For this review, take the finished solid that the model builds, in its own axes (mm). Face numbers are marked on the shaded views. A direction names the side the tool comes from. Round coordinates to 2 decimals unless told otherwise and drop trailing zeros. Order: outer loops, then holes, each group sorted by start corner. A loop starts at its lowest first (then second) coordinate and runs counter-clockwise, first axis right, second up. Notation, with made-up numbers: (1, -13.75) - (27, -13.75) arc R25 ccw to (27, 8.25) - close; hole circle Ø8 at (-13, 57). An arc over 180 degrees is marked (long way). Write each question's results on one line, items separated by ' | '. Start each with the question number.
(1) Draft analysis for pull direction X (two halves, no side actions). For the marked faces 5, 6 and 7, state which applies: pulls with the +X half, pulls with the -X half, needs draft (parallel to the pull), parting line crosses it, or undercut.
(2) For L1, parallel to Y at x = 5.5, z = 1.75; L2, parallel to Z at x = -11.5, y = -2; L3, parallel to Y at x = 11.7, z = 1.1, list the stretches that pass through material, from the lowest coordinate up. Write a range as from..to.
(3) Take a section at A-A, the plane z = 6. Give the boundary of the cut face in (x, y).
(4) Take a section at B-B, the plane x = -1.75. Give the boundary of the cut face in (y, z).
(5) Insertion check: pin 1 Ø4.5 at (x, y) = (-12, 2.5) entering from +Z; pin 2 Ø2 at (x, z) = (5.5, 10.5) entering from -Y; pin 3 Ø5.5 at (x, y) = (-6, -0.5) entering from -Z. Each pin has a flat end and moves straight along its axis. Give the tip position at first contact, or say it passes through.
(6) For the marked faces 1, 2, 3 and 4, list the 3-axis set-ups (+Z, -Z, +X, -X, +Y, -Y) from which the entire face can be reached by the end or side of a thin tool; tool diameter is ignored.
(7) Take a section at D-D, the plane z = -2. Give the boundary of the cut face in (x, y) (3 decimals), plus the area to 3 significant figures.
```python
from build123d import *

# Parameters (mm, degrees)
ESQUISSE1_W             = 27
ESQUISSE1_H             = 10.8
BOSS_EXTRU_1_DEPTH      = 8
ESQUISSE2_R             = 1.05
ENL_V_MAT_EXTRU_1_DEPTH = 17.595481313
ESQUISSE3_W             = 19.2
ESQUISSE3_H             = 8
BOSS_EXTRU_2_DEPTH      = 4
ENL_V_MAT_EXTRU_2_DEPTH = 6.5
ESQUISSE5_W             = 4
ESQUISSE5_H             = 6
ESQUISSE5_R             = 1
ESQUISSE5_W_2           = 10.7
ENL_V_MAT_EXTRU_3_DEPTH = 1
ESQUISSE6_W             = 9.85
ESQUISSE6_H             = 1.4
ENL_V_MAT_EXTRU_4_DEPTH = 17.595481313
ESQUISSE7_W             = 6
ESQUISSE7_H             = 6
BOSS_EXTRU_3_DEPTH      = 3.5
ESQUISSE8_W             = 5
ESQUISSE8_H             = 2.5
ENL_V_MAT_EXTRU_5_DEPTH = 3.5
ENL_V_MAT_EXTRU_6_DEPTH = 2


with BuildPart() as part:
    # Esquisse1 → Boss.-Extru.1 (new body)
    with BuildSketch(Plane.XY):
        Rectangle(ESQUISSE1_W, ESQUISSE1_H)
    extrude(amount=BOSS_EXTRU_1_DEPTH)

    # Esquisse2 → Enlèv. mat.-Extru.1 (cut, through all)
    with BuildSketch(Plane.XY.offset(8)):
        with Locations((-11.7, 3.3)):
            Circle(ESQUISSE2_R)
        with Locations((11.7, -3.3)):
            Circle(ESQUISSE2_R)
    extrude(amount=-ENL_V_MAT_EXTRU_1_DEPTH, mode=Mode.SUBTRACT)

    # Esquisse3 → Boss.-Extru.2 (add)
    with BuildSketch(Plane.XY.offset(8)):
        Rectangle(ESQUISSE3_W, ESQUISSE3_H)
    extrude(amount=BOSS_EXTRU_2_DEPTH)

    # Esquisse4 → Enlèv. mat.-Extru.2 (cut)
    with BuildSketch(Plane.XY.offset(8)):
        with BuildLine():
            Line((-9.6, 3.7), (-9.6, 5.4))
            Line((-9.6, 5.4), (-13.5, 5.4))
            Line((-13.5, 5.4), (-13.5, 1.5))
            Line((-13.5, 1.5), (-11.8, 1.5))
            ThreePointArc((-11.8, 1.5), (-10.244365081, 2.144365081), (-9.6, 3.7))
        make_face()
        with BuildLine():
            Line((9.6, -5.4), (13.5, -5.4))
            Line((13.5, -5.4), (13.5, -1.5))
            Line((13.5, -1.5), (11.8, -1.5))
            ThreePointArc((11.8, -1.5), (10.244365081, -2.144365081), (9.6, -3.7))
            Line((9.6, -3.7), (9.6, -5.4))
        make_face()
    extrude(amount=-ENL_V_MAT_EXTRU_2_DEPTH, mode=Mode.SUBTRACT)

    # Esquisse5 → Enlèv. mat.-Extru.3 (cut)
    # profile 1 of 2: a face of its own
    with BuildSketch(Plane.XY.offset(12)):
        with Locations((-6.1, 0)):
            Rectangle(ESQUISSE5_W, ESQUISSE5_H)
        with Locations((-6.1, 0)):
            Circle(ESQUISSE5_R, mode=Mode.SUBTRACT)
    # profile 2 of 2: a face of its own
    with BuildSketch(Plane.XY.offset(12)):
        with Locations((2.75, 0)):
            Rectangle(ESQUISSE5_W_2, ESQUISSE5_H)
        with Locations((5.78, 0)):
            Circle(ESQUISSE5_R, mode=Mode.SUBTRACT)
    extrude(amount=-ENL_V_MAT_EXTRU_3_DEPTH, mode=Mode.SUBTRACT)

    # Esquisse6 → Enlèv. mat.-Extru.4 (cut, through all)
    with BuildSketch(Plane.XY.offset(8)):
        with Locations((-8.575, -4.7)):
            Rectangle(ESQUISSE6_W, ESQUISSE6_H)
    extrude(amount=-ENL_V_MAT_EXTRU_4_DEPTH, mode=Mode.SUBTRACT)

    # Esquisse7 → Boss.-Extru.3 (add)
    with BuildSketch(Plane.XZ.offset(4)):
        with Locations((-8.575, 0)):
            Rectangle(ESQUISSE7_W, ESQUISSE7_H)
    extrude(amount=BOSS_EXTRU_3_DEPTH)

    # Esquisse8 → Enlèv. mat.-Extru.5 (cut)
    with BuildSketch(Plane(origin=(0, 0, -3), x_dir=(-1, 0, 0), z_dir=(0, 0, -1))):
        with Locations((8.575, -5.75)):
            Rectangle(ESQUISSE8_W, ESQUISSE8_H)
    extrude(amount=-ENL_V_MAT_EXTRU_5_DEPTH, mode=Mode.SUBTRACT)

    # Esquisse9 → Enlèv. mat.-Extru.6 (cut)
    with BuildSketch(Plane(origin=(0, 0, 0), x_dir=(-1, 0, 0), z_dir=(0, 0, -1))):
        with BuildLine():
            Line((9, 4.9), (-13, 4.9))
            Line((-13, 4.9), (-13, -0.9))
            ThreePointArc((-13, -0.9), (-10.171572875, -2.071572875), (-9, -4.9))
            Line((-9, -4.9), (3.65, -4.9))
            Line((3.65, -4.9), (3.65, -4))
            Line((3.65, -4), (13, -4))
            Line((13, -4), (13, 0.9))
            ThreePointArc((13, 0.9), (10.171572875, 2.071572875), (9, 4.9))
        make_face()
    extrude(amount=-ENL_V_MAT_EXTRU_6_DEPTH, mode=Mode.SUBTRACT)


solid = part.part
```
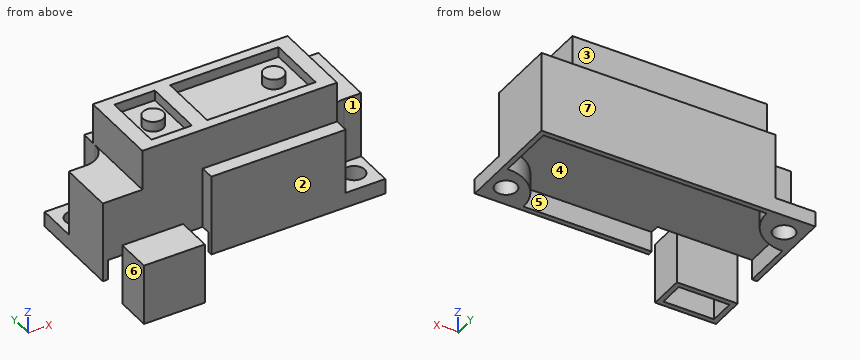
Results below:
1) face 5: undercut | face 6: pulls with the -X half | face 7: needs draft
2) L1: y = -5.4..-4.9, 4.9..5.4 | L2: z = 2..8 | L3: y = -5.4..-4.35, -2.25..-1.12, 4.9..5.4
3) outline: (-13.5, -4) - (-3.65, -4) - (-3.65, -5.4) - (9.6, -5.4) - (9.6, -3.7) arc R2.2 cw to (11.8, -1.5) - (13.5, -1.5) - (13.5, 5.4) - (-9.6, 5.4) - (-9.6, 3.7) arc R2.2 cw to (-11.8, 1.5) - (-13.5, 1.5) - close
4) outline: (-5.4, 0) - (-4.9, 0) - (-4.9, 2) - (4.9, 2) - (4.9, 0) - (5.4, 0) - (5.4, 8) - (4, 8) - (4, 12) - (3, 12) - (3, 11) - (-3, 11) - (-3, 12) - (-4, 12) - (-4, 8) - (-5.4, 8) - close
5) pin 1: stops at z = 8 | pin 2: stops at y = -4 | pin 3: stops at z = 2
6) face 1: +Z, +X, -Y | face 2: +Z, -Z, +X, -Y | face 3: +Z, +X, -X, +Y | face 4: -Z
7) outline: (-11.575, -7.5) - (-5.575, -7.5) - (-5.575, -4) - (-11.575, -4) - close; hole (-11.075, -7) - (-6.075, -7) - (-6.075, -4.5) - (-11.075, -4.5) - close | area: 8.50 mm^2
